Autodesk Inventor part; units mm, degrees
ref_plane "YZ Plane" through (0, 0, 0) normal (1, 0, 0) x (0, 1, 0)
ref_plane "XZ Plane" through (0, 0, 0) normal (0, 1, 0) x (-1, 0, 0)
ref_plane "XY Plane" through (0, 0, 0) normal (0, 0, 1) x (1, 0, 0)
sketch "Sketch1" plane through (0, 0, 0) normal (0, 0, 1) x (1, 0, 0)
  line L0 (-245, -275) -> (245, -275)
  line L1 (245, -275) -> (245, 275)
  line L2 (245, 275) -> (-245, 275)
  line L3 (-245, 275) -> (-245, -275)
  line L4 (-245, -275) -> (245, 275) construction
  line L5 (245, -275) -> (-245, 275) construction
  line L6 (-245, 265) -> (245, 265) construction
  line L7 (-235, 275) -> (-235, -275) construction
  line L8 (235, 275) -> (235, -275) construction
  line L9 (-245, -165) -> (245, -165) construction
  line L10 (-245, 195) -> (245, 195) construction
  circle A0 centre (-235, 265) radius 2.1
  circle A1 centre (-135, 265) radius 2.1
  circle A2 centre (135, 265) radius 2.1
  circle A3 centre (235, 265) radius 2.1
  circle A4 centre (135, 195) radius 2.1
  circle A5 centre (235, 195) radius 2.1
  circle A6 centre (-235, 195) radius 2.1
  circle A7 centre (-135, 195) radius 2.1
  line L11 (-135, 275) -> (-135, -275) construction
  line L12 (0, 0) -> (0, -275) construction
  line L13 (135, 275) -> (135, -275) construction
  circle A8 centre (-235, 70) radius 2.1
  circle A9 centre (135, -165) radius 2.1
  circle A10 centre (-135, -165) radius 2.1
  circle A11 centre (-235, -70) radius 2.1
  circle A12 centre (-235, -220) radius 2.1
  circle A13 centre (235, -220) radius 2.1
  circle A14 centre (235, -70) radius 2.1
  circle A15 centre (235, 70) radius 2.1
  line L14 (-235, 70) -> (235, 70) construction
  line L15 (-235, -70) -> (235, -70) construction
  line L16 (-235, 0) -> (235, 0) construction
  line L17 (-235, -220) -> (235, -220) construction
  line L18 (0, 275) -> (0, 0) construction
  circle A16 centre (0, 265) radius 2.1
  circle A17 centre (0, 195) radius 2.1
  circle A18 centre (0, -165) radius 2.1
  line L19 (143, 138) -> (185, 138) construction
  line L20 (185, 138) -> (185, 180) construction
  line L21 (185, 180) -> (143, 180) construction
  line L22 (143, 180) -> (143, 138) construction
  line L23 (143, 138) -> (185, 180) construction
  line L24 (185, 138) -> (143, 180) construction
  circle A19 centre (164, 159) radius 11
  line L25 (148.5, 143.5) -> (179.5, 143.5) construction
  line L26 (179.5, 143.5) -> (179.5, 174.5) construction
  line L27 (179.5, 174.5) -> (148.5, 174.5) construction
  line L28 (148.5, 174.5) -> (148.5, 143.5) construction
  line L29 (148.5, 143.5) -> (179.5, 174.5) construction
  line L30 (179.5, 143.5) -> (148.5, 174.5) construction
  circle A20 centre (148.5, 174.5) radius 1.7
  circle A21 centre (179.5, 174.5) radius 1.7
  circle A22 centre (179.5, 143.5) radius 1.7
  circle A23 centre (148.5, 143.5) radius 1.7
  dimension "d0" = 490
  dimension "d1" = 550
  dimension "d2" = 10
  dimension "d3" = 10
  dimension "d4" = 10
  dimension "d5" = 110
  dimension "d6" = 80
  dimension "d7" = 110
  dimension "d8" = 110
  dimension "d9" = 70
  dimension "d10" = 55
  dimension "d11" = 4.2
  dimension "d14" = 42
  dimension "d15" = 15
  dimension "d16" = 50
  dimension "d17" = 31
  dimension "d18" = 3.4
  dimension "d19" = 22
extrude "Plate3" add sketch "Sketch1" along normal blind 1.5
sketch "Sketch2" plane through (0, 0, 1.5) normal (0, 0, 1) x (1, 0, 0)
  line L0 (-200, 215.5) -> (200, 215.5) construction
  line L1 (-200, 205.5) -> (200, 205.5)
  line L2 (200, 225.5) -> (-200, 225.5)
  arc A0 (-200, 225.5) -> (-200, 205.5) centre (-200, 215.5) ccw
  arc A1 (200, 205.5) -> (200, 225.5) centre (200, 215.5) ccw
  circle A2 centre (0, 195) radius 2.1 construction
  circle A3 centre (0, 265) radius 2.1 construction
  line L3 (0, 195) -> (0, 215.5) construction
  point P0 (0, 0)
  dimension "d23" = 20
  dimension "d24" = 400
  dimension "d28" = 10.5
extrude "Cut1" cut sketch "Sketch2" against normal blind 1.5
equation "\"d25\" = Thickness"
equation "\"d21\" = Thickness"
equation "\"CornerReliefSize\" = 4 * Thickness"
equation "\"TransitionRadius\" = BendRadius"
equation "\"JacobiRadiusSize\" = BendRadius"
equation "\"d12\" = BendRadius"
equation "\"d13\" = BendRadius"
equation "\"d20\" = BendRadius"
properties part number "Side Cladding" material "Aluminium 1050"
The model under review builds one solid part; all positions refer to its coordinate system, in mm. Coordinates: 2 decimals unless noted, no trailing zeros. Write each loop counter-clockwise with the first axis right and the second up, starting at its lowest first coordinate (ties: lowest second). Pieces come first, ordered by that corner, then holes. Notation, with made-up numbers: (-30.75, -37.75) -> (0.25, -37.75) arc R28 ccw to (0.25, -1.75) -> close; hole circle Ø1 at (34, 79.25). An arc over 180 degrees is marked (long way). One line per item, written item: value. Start each with the question number.
Q1. Clearance check with flat-ended pins moving along their axes: P1, Ø4, axis at x = 235, y = -220, coming from the +Z side (3 decimals); P2, Ø5, axis at x = -135, y = -165, coming from the -Z side. State where each tip first meets the part, or that it passes through.
Q2. Add section C-C, the plane x = -148. Give the boundary of the cut face in (y, z), then the cut area to 3 significant figures.
Q3. Add section B-B, the plane y = 215.5. Give the boundary of the cut face in (x, z), then the cut area to 3 significant figures.
Q4. To check wall thickness, follow probe 1 along Y at (x, z) = (-135, 0.3); probe 2 along X at (y, z) = (195, 0.45); probe 3 along Y at (x, z) = (-235, 1.25). State the ranges of each line that lie inside material, in increasing order.
Q5. Add section A-A, the plane z = 0.25. Count the separate pieces of the cut face and the enclosed holes in it, then the cut area to 3 significant figures.
Q6. The part is to be moulded in two halves that separate along X. For faces 1 (the face through (-3, 4, 0)), 2 (the face through (155.89, 151.57, 0.74)), say which applies: +X half, -X half, draft (parallel to the pull), parting line (faces both ways), or undercut.
Response:
1. P1: through
1. P2: z = 0
2. outline: (-275, 0) -> (205.5, 0) -> (205.5, 1.5) -> (-275, 1.5) -> close; (225.5, 0) -> (275, 0) -> (275, 1.5) -> (225.5, 1.5) -> close
2. area: 795 mm²
3. outline: (-245, 0) -> (-210, 0) -> (-210, 1.5) -> (-245, 1.5) -> close; (210, 0) -> (245, 0) -> (245, 1.5) -> (210, 1.5) -> close
3. area: 105 mm²
4. probe 1: -275 to -167.1, -162.9 to 192.9, 197.1 to 205.5, 225.5 to 262.9, 267.1 to 275
4. probe 2: -245 to -237.1, -232.9 to -137.1, -132.9 to -2.1, 2.1 to 132.9, 137.1 to 232.9, 237.1 to 245
4. probe 3: -275 to -222.1, -217.9 to -72.1, -67.9 to 67.9, 72.1 to 192.9, 197.1 to 262.9, 267.1 to 275
5. separate pieces: 1
5. enclosed holes: 25
5. area: 261,000 mm²
6. face 1: draft
6. face 2: undercut
